Source: CAD feature listing. Evaluate the final solid. Frame: model axes, mm. A direction names the side the tool comes from. Give positions to 0.01 mm unless a question says otherwise; leave off trailing zeros. Loops run counter-clockwise (first coordinate to the right, second up) from the corner with the lowest first, then second, coordinate; pieces in that order, holes last. Notation, with made-up numbers: M 18.5,63.5 L 63.5,63.5 A16 ccw 63.5,74.5 Z; hole C 4,69 d2. An arc over 180 degrees is marked long. Answer in a Markdown table with one row per item.
```python
from build123d import *

# Parameters (mm, degrees)
SKETCH1_W                    = 50
SKETCH1_H                    = 7
REVOLVE5_ANGLE               = 167.5
SHELL2_T                     = 3
CUT_EXTRUDE3_DEPTH           = 77.072333999
CUT_EXTRUDE3_DEPTH_BACK      = 10
CUT_EXTRUDE4_DEPTH           = 77.072333999
CUT_EXTRUDE4_DEPTH_BACK      = 10
CUT_EXTRUDE_THIN1_DEPTH      = 77.072333999
CUT_EXTRUDE_THIN1_DEPTH_BACK = 20
CUT_EXTRUDE_THIN2_DEPTH      = 77.072333999
CUT_EXTRUDE_THIN2_DEPTH_BACK = 20
CUT_EXTRUDE_THIN3_DEPTH      = 76.000787866
CUT_EXTRUDE_THIN3_DEPTH_BACK = 20
SKETCH18_R                   = 8
BOSS_EXTRUDE3_DEPTH          = 3
SKETCH22_W                   = 13
SKETCH22_H                   = 12.488136332
BOSS_EXTRUDE4_DEPTH          = 1
SKETCH23_W                   = 13
SKETCH23_H                   = 12.478928716
BOSS_EXTRUDE5_DEPTH          = 1
CUT_EXTRUDE_THIN4_DEPTH      = 76.647331154
CUT_EXTRUDE_THIN4_DEPTH_BACK = 20
CUT_EXTRUDE_THIN5_DEPTH      = 76.000787866
CUT_EXTRUDE_THIN5_DEPTH_BACK = 20


with BuildPart() as part:
    # Sketch1 → Revolve5 (revolve)
    with BuildSketch(Plane(origin=(0, 0, 0), x_dir=(1, 0, 0), z_dir=(0, 1, 0))):
        with Locations((25, 3.5)):
            Rectangle(SKETCH1_W, SKETCH1_H)
    revolve(axis=Axis((0, 0, 0), (0, 0, 1)), revolution_arc=REVOLVE5_ANGLE)

    # Shell2
    shell2_openings = [part.faces().sort_by_distance(p)[0] for p in [
        (25, 0, -3.5),
        (-24.407400178, 5.410990348, -3.5),
    ]]
    offset(amount=SHELL2_T, openings=shell2_openings, kind=Kind.INTERSECTION)

    # Sketch11 → Cut-Extrude3 (cut, two sides: drawn at the far end of the back side and taken through both)
    with BuildSketch(Plane.XY.offset(3).offset(-CUT_EXTRUDE3_DEPTH_BACK)):
        Polygon((-295.067343662, 38.119573796), (-51.743688377, 11.471299539), (53, 0), (296.323655284, -26.648274258), (243.027106769, -513.295584826), (-348.363892177, -448.527736772), align=None)
    extrude(amount=CUT_EXTRUDE3_DEPTH + CUT_EXTRUDE3_DEPTH_BACK, mode=Mode.SUBTRACT)

    # Sketch12 → Cut-Extrude4 (cut, two sides: drawn at the far end of the back side and taken through both)
    with BuildSketch(Plane(origin=(0, 0, -10), x_dir=(-1, 0, 0), z_dir=(0, 0, -1)).offset(-CUT_EXTRUDE4_DEPTH_BACK)):
        Polygon((-296.323655284, -26.648274258), (-53, 0), (51.743688377, 11.471299539), (295.067343662, 38.119573796), (348.363892177, -448.527736772), (-243.027106769, -513.295584826), align=None)
    extrude(amount=CUT_EXTRUDE4_DEPTH + CUT_EXTRUDE4_DEPTH_BACK, mode=Mode.SUBTRACT)

    # Sketch13 → Cut-Extrude-Thin1 (cut, two sides: drawn at the far end of the back side and taken through both)
    with BuildSketch(Plane(origin=(0, 0, -10), x_dir=(-1, 0, 0), z_dir=(0, 0, -1)).offset(-CUT_EXTRUDE_THIN1_DEPTH_BACK)):
        Polygon((48.779244367, 11.146640118), (47.419699991, 23.560551191), (57.360263374, 24.64921994), (58.719807749, 12.235308866), align=None)
    extrude(amount=CUT_EXTRUDE_THIN1_DEPTH + CUT_EXTRUDE_THIN1_DEPTH_BACK, mode=Mode.SUBTRACT)

    # Sketch14 → Cut-Extrude-Thin2 (cut, two sides: drawn at the far end of the back side and taken through both)
    with BuildSketch(Plane(origin=(0, 0, -10), x_dir=(-1, 0, 0), z_dir=(0, 0, -1)).offset(-CUT_EXTRUDE_THIN2_DEPTH_BACK)):
        Polygon((-50.035555989, 0.324659421), (-51.39409796, 12.729417605), (-81.215788107, 9.46341136), (-79.857246136, -2.941346825), align=None)
    extrude(amount=CUT_EXTRUDE_THIN2_DEPTH + CUT_EXTRUDE_THIN2_DEPTH_BACK, mode=Mode.SUBTRACT)

    # Sketch15 → Cut-Extrude-Thin3 (cut, two sides: drawn at the far end of the back side and taken through both)
    with BuildSketch(Plane(origin=(0, 0, -10), x_dir=(-1, 0, 0), z_dir=(0, 0, -1)).offset(-CUT_EXTRUDE_THIN3_DEPTH_BACK)):
        with BuildLine():
            ThreePointArc((-41.982664634, 1.20659446), (-4.572408744, 41.750366205), (40.726353012, 10.264705079))
            Line((40.726353012, 10.264705079), (11.636100861, 2.93277288))
            ThreePointArc((11.636100861, 2.93277288), (-1.306402498, 11.928676059), (-11.995047038, 0.344741274))
            Line((-11.995047038, 0.344741274), (-41.982664634, 1.20659446))
        make_face()
    extrude(amount=CUT_EXTRUDE_THIN3_DEPTH + CUT_EXTRUDE_THIN3_DEPTH_BACK, mode=Mode.SUBTRACT)


with BuildPart() as body_2:
    # of the pieces the cut leaves, the one that is kept (cut_extrude_thin3_keep)
    add(part.part.solids().sort_by_distance((49.998919737, 0.328671743, 0))[0])

    # Sketch18 → Boss-Extrude3 (add)
    with BuildSketch(Plane.XY.offset(3)):
        with Locations((-39.855418013, 18.217155785)):
            Circle(SKETCH18_R)
        with Locations((42.853599633, 9.159045166)):
            Circle(SKETCH18_R)
    extrude(amount=-BOSS_EXTRUDE3_DEPTH)

    # Sketch22 → Boss-Extrude4 (add)
    with BuildSketch(Plane(origin=(-49.407400178, 5.410990348, 0), x_dir=(0, 0, 1), z_dir=(-0.99405633822232, 0.10886687485196148, 0))):
        with Locations((-3.5, 12.014012533)):
            Rectangle(SKETCH22_W, SKETCH22_H)
    extrude(amount=BOSS_EXTRUDE4_DEPTH)

    # Sketch23 → Boss-Extrude5 (add)
    with BuildSketch(Plane(origin=(49.407400178, -5.410990348, 0), x_dir=(0, 0, -1), z_dir=(0.9940563382223201, -0.10886687485196078, 0))):
        with Locations((3.5, 12.009408725)):
            Rectangle(SKETCH23_W, SKETCH23_H)
    extrude(amount=BOSS_EXTRUDE5_DEPTH)

    # Sketch25 → Cut-Extrude-Thin4 (cut, two sides: drawn at the far end of the back side and taken through both)
    with BuildSketch(Plane(origin=(0, 0, -10), x_dir=(-1, 0, 0), z_dir=(0, 0, -1)).offset(-CUT_EXTRUDE_THIN4_DEPTH_BACK)):
        Polygon((-51.450152385, 12.723278647), (-51.029612328, 0.215792546), (-61.023964562, -0.12024824), (-61.44450462, 12.387237861), align=None)
    extrude(amount=CUT_EXTRUDE_THIN4_DEPTH + CUT_EXTRUDE_THIN4_DEPTH_BACK, mode=Mode.SUBTRACT)

    # Sketch26 → Cut-Extrude-Thin5 (cut, two sides: drawn at the far end of the back side and taken through both)
    with BuildSketch(Plane.XY.offset(3).offset(-CUT_EXTRUDE_THIN5_DEPTH_BACK)):
        Polygon((-47.472396692, 23.566322419), (-49.773300705, 11.255506993), (-59.603087399, 13.092704194), (-57.302183385, 25.40351962), align=None)
    extrude(amount=CUT_EXTRUDE_THIN5_DEPTH + CUT_EXTRUDE_THIN5_DEPTH_BACK, mode=Mode.SUBTRACT)


solid = body_2.part
```
1) Material intervals for L1, parallel to Z at x = 41.5, y = 13.5; L2, parallel to X at y = 27, z = -4.25; L3, parallel to X at y = 23, z = -1.25, sorted ascending.
Reply:
| item | result |
|---|---|
| L1 | z = -10 to -7, 0 to 3 |
| L2 | x = -45.61 to -42.08, 42.08 to 45.61 |
| L3 | x = -47.58 to -44.4, 44.4 to 47.75 |
2) Pull-direction query (X, two-part tool) for faces 4 (the flat face through (8, 43, -10)), 5 (the flat face through (5, 44, -7)), 6 (the flat face through (-48.607, 17.497, -3.591)), 7 (the cylindrical face through (6.67, 52.58, -3.59)); classes: released by +X, released by -X, zero draft, split by the parting line, or undercut.
Reply:
| item | result |
|---|---|
| face 4 | zero draft |
| face 5 | undercut |
| face 6 | released by -X |
| face 7 | split by the parting line |
3) Section A-A, the plane z = 1. Return loops of the section in (x, y), then the cut area to 3 significant figures.
Reply:
| item | result |
|---|---|
| outline | M -49.77,11.26 L -40.73,10.26 A8 ccw -34.41,24.08 A42 cw 38.81,16.06 A8 ccw 41.98,1.21 L 51.03,0.22 L 51.45,12.72 A53 ccw -47.47,23.57 Z |
| area | 1,620 mm² |
4) Section D-D, the plane y = 27. Return loops of the section in (x, z).
Reply:
| item | result |
|---|---|
| outline | M -45.61,-10 L -32.17,-10 L -32.17,-7 L -42.08,-7 L -42.08,0 L -32.17,0 L -32.17,3 L -45.61,3 Z; M 32.17,-10 L 45.61,-10 L 45.61,3 L 32.17,3 L 32.17,0 L 42.08,0 L 42.08,-7 L 32.17,-7 Z |
5) Section C-C, the plane x = -22.5. Return loops of the section in (y, z), then the cut area to 3 significant figures.
Reply:
| item | result |
|---|---|
| outline | M 35.46,-10 L 47.99,-10 L 47.99,3 L 35.46,3 L 35.46,0 L 44.65,0 L 44.65,-7 L 35.46,-7 Z |
| area | 98.5 mm² |
6) Pin query (flat end, axial travel): pin 1 Ø6 at (x, z) = (-16.5, -1) entering from +Y; pin 2 Ø4 at (x, z) = (9.5, -3) entering from -Y; pin 3 Ø4 at (y, z) = (30.5, -7) entering from -X (3 decimals). Return the tip coordinate at first contact, or that it passes through.
Reply:
| item | result |
|---|---|
| pin 1 | stops at y = 51.25 |
| pin 2 | stops at y = 48.66 |
| pin 3 | stops at x = -44.685 |
7) Section B-B, the plane y = 33.5. Return loops of the section in (x, z), then the cut area to 3 significant figures.
Reply:
| item | result |
|---|---|
| outline | M -41.07,-10 L -25.33,-10 L -25.33,-7 L -37.12,-7 L -37.12,0 L -25.33,0 L -25.33,3 L -41.07,3 Z; M 25.33,-10 L 41.07,-10 L 41.07,3 L 25.33,3 L 25.33,0 L 37.12,0 L 37.12,-7 L 25.33,-7 Z |
| area | 244 mm² |
8) Set-up query: faces 1 (the cylindrical face through (-32.64, 14.76, 1.52)), 2 (the cylindrical face through (5.41, 41.65, -8.48)), 3 (the flat face through (4, 42, 0)). Return all of +Z, -Z, +X, -X, +Y, -Y with unobstructed straight access to the full face (end or side cutting, diameter ignored); none if empty.
Reply:
| item | result |
|---|---|
| face 1 | +Z, -Z |
| face 2 | -Z, -Y |
| face 3 | -Y |
